Geometry: final body of the model. Coordinates: model frame, mm. Face numbers are marked on the shaded views. A direction names the side the tool comes from. Give positions to 0.01 mm unless a question says otherwise; leave off trailing zeros. Write each loop counter-clockwise with the first axis right and the second up, starting at its lowest first coordinate (ties: lowest second). Pieces come first, ordered by that corner, then holes.
from build123d import *

# Parameters (mm, degrees)
SKETCH1_R           = 5.6
BOSS_EXTRUDE1_DEPTH = 33.67
SKETCH2_R           = 11.885
SKETCH3_R           = 12.675
FILLET1_R           = 3
CHAMFER1_SIZE       = 0.8
CHAMFER1_SIZE2      = 9
FILLET2_R           = 3


# Read off the part's stored shape, not the designer's step: Shell1
with BuildPart() as part:
    # Sketch1 → Boss-Extrude1 (new body)
    with BuildSketch(Plane(origin=(0, 0, 0), x_dir=(1, 0, 0), z_dir=(0, 1, 0))):
        with Locations(Location((0, 0, 0), (0, 0, 270))):
            Circle(SKETCH1_R)
    extrude(amount=BOSS_EXTRUDE1_DEPTH)

    # Sketch2 → Loft1 section 0
    with BuildSketch(Plane(origin=(0, 33.67, 0), x_dir=(1, 0, 0), z_dir=(0, 1, 0))):
        Circle(SKETCH2_R)
    # Sketch3 → Loft1 section 1
    with BuildSketch(Plane(origin=(0, 46.03, 0), x_dir=(1, 0, 0), z_dir=(0, 1, 0))):
        Circle(SKETCH3_R)
    loft()

    # Shell1 outline → Shell1 (revolve, cut)
    with BuildSketch(Plane.XY):
        Polygon((0, 46.03), (0, 34.87), (10.759250385, 34.87), (11.472551356, 46.03), align=None)
    revolve(axis=Axis((0, 0, 0), (0, 1, 0)), mode=Mode.SUBTRACT)

    # Fillet1
    fillet1_edges = [part.edges().sort_by_distance(p)[0] for p in [
        (-11.885, 33.67, 0),
    ]]
    fillet(fillet1_edges, radius=FILLET1_R)

    # Chamfer1
    chamfer1_edges = [part.edges().sort_by_distance(p)[0] for p in [
        (-11.472551356, 46.03, 0),
    ]]
    chamfer1_side = [part.faces().sort_by_distance(p)[0] for p in [
        (-12.316496862, 46.03, 0),
    ]]
    chamfer(chamfer1_edges, length=CHAMFER1_SIZE, length2=CHAMFER1_SIZE2, reference=chamfer1_side[0])

    # Fillet2
    fillet2_edges = [part.edges().sort_by_distance(p)[0] for p in [
        (-10.759250385, 34.87, 0),
    ]]
    fillet(fillet2_edges, radius=FILLET2_R)


solid = part.part
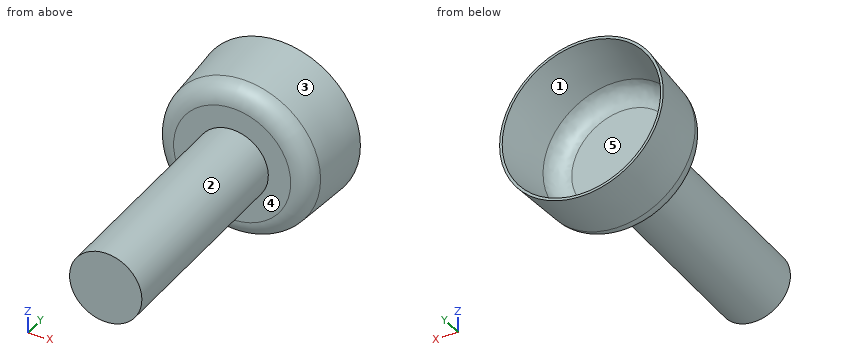
Q1. Access query for the marked faces 1 and 2. Directions: +Z, -Z, +X, -X, +Y, -Y. A direction counts if a zero-diameter tool reaches every point of the face in a straight line with its end or side. Return the directions, or none.
Filled sheet:
face 1: +Y
face 2: -Y
Q2. Pin query (flat end, axial travel): P1, Ø5, axis at x = 7.5, y = 29, coming from the -Z side; P2, Ø8, axis at x = -1, z = 2.5, coming from the +Y side; P3, Ø6, axis at x = -1, y = 27, coming from the +Z side. Return the tip coordinate at first contact, or that it passes through.
Filled sheet:
P1: stops at z = -2.52
P2: stops at y = 34.87
P3: stops at z = 5.6
Q3. Pull-direction query (X, two-part tool) for the marked faces 3, 4 and 5; classes: released by +X, released by -X, zero draft, split by the parting line, or undercut.
Filled sheet:
face 3: split by the parting line
face 4: zero draft
face 5: undercut
Q4. Ray query, line 1 along Y through (x, z) = (-3, -4.5); line 2 along X through (y, z) = (37, 8.5); line 3 along Z through (x, y) = (3.5, 37.5). Return the intervals inside material, ascending.
Filled sheet:
line 1: y = 0 to 34.87
line 2: x = -8.61 to -6.76, 6.76 to 8.61
line 3: z = -11.61 to -10.39, 10.39 to 11.61
Q5. Section A-A on y = 28. Output: boundary loops of the cut face in (x, z).
Filled sheet:
outline: circle Ø11.2 at (0, 0)
